Verification items for the finished model (mm, model axes). Face numbers are marked on the shaded views. A direction names the side the tool comes from. Round coordinates to 2 decimals unless told otherwise and drop trailing zeros. Order: outer loops, then holes, each group sorted by start corner. A loop starts at its lowest first (then second) coordinate and runs counter-clockwise, first axis right, second up. Notation, with made-up numbers: (74, 34) -> (132, 34) arc R31 cw to (132, 65) -> close; hole circle Ø6 at (26, -33). An arc over 180 degrees is marked (long way). Write item = value, one per line. Start each with the question number.
from build123d import *

# Parameters (mm, degrees)
SKETCH1_W                  = 68.6
SKETCH1_H                  = 20.38979341
BRACKETBASE_DEPTH          = 5
SKETCH2_W                  = 20.38979341
SKETCH2_H                  = 12
LEGMOUNTINGTAB_DEPTH       = 5
SKETCH3_R                  = 2
LEGMOUNTINGHOLES_DEPTH     = 5
SKETCH4_W                  = 20.38979341
SKETCH4_H                  = 7
ARDUINOMOUNTINGTAB_DEPTH   = 4.38979341
SKETCH5_R                  = 2
ARDUINOMOUNTINGHOLES_DEPTH = 5
FILLET1_R                  = 2


with BuildPart() as part:
    # Sketch1 → bracketBase (new body)
    with BuildSketch(Plane(origin=(0, 0, 0), x_dir=(1, 0, 0), z_dir=(0, 1, 0))):
        with Locations((34.3, 10.194896705)):
            Rectangle(SKETCH1_W, SKETCH1_H)
    extrude(amount=BRACKETBASE_DEPTH)

    # Sketch2 → legMountingTab (add)
    with BuildSketch(Plane.ZY):
        with Locations((-10.194896705, 6)):
            Rectangle(SKETCH2_W, SKETCH2_H)
    legmountingtab = extrude(amount=-LEGMOUNTINGTAB_DEPTH)

    # Sketch3 → legMountingHoles (cut)
    with BuildSketch(Plane(origin=(5, 0, 0), x_dir=(0, 0, -1), z_dir=(1, 0, 0))):
        with Locations((15.13979341, 8.75)):
            Circle(SKETCH3_R)
        with Locations((5.13979341, 8.75)):
            Circle(SKETCH3_R)
    legmountingholes = extrude(amount=-LEGMOUNTINGHOLES_DEPTH, mode=Mode.SUBTRACT)

    # legMountingHoles2: legMountingTab, legMountingHoles across plane
    add(legmountingtab.mirror(Plane.ZY.offset(-34.3)))
    add(legmountingholes.mirror(Plane.ZY.offset(-34.3)), mode=Mode.SUBTRACT)

    # Sketch4 → arduinoMountingTab (add)
    with BuildSketch(Plane.XY):
        with Locations((34.3, -3.5)):
            Rectangle(SKETCH4_W, SKETCH4_H)
    extrude(amount=-ARDUINOMOUNTINGTAB_DEPTH)

    # Sketch5 → arduinoMountingHoles (cut)
    with BuildSketch(Plane.XY):
        with Locations((39.397448352, -3.5)):
            Circle(SKETCH5_R)
        with Locations(Location((29.202551647, -3.5, 0), (0, 0, 180))):
            Circle(SKETCH5_R)
    extrude(amount=-ARDUINOMOUNTINGHOLES_DEPTH, mode=Mode.SUBTRACT)

    # Fillet1
    fillet1_edges = [part.edges().sort_by_distance(p)[0] for p in [
        (44.494896705, 0, -2.194896705),
        (44.494896705, -7, -2.194896705),
        (24.105103295, -7, -2.194896705),
        (24.105103295, 0, -2.194896705),
    ]]
    fillet(fillet1_edges, radius=FILLET1_R)


solid = part.part
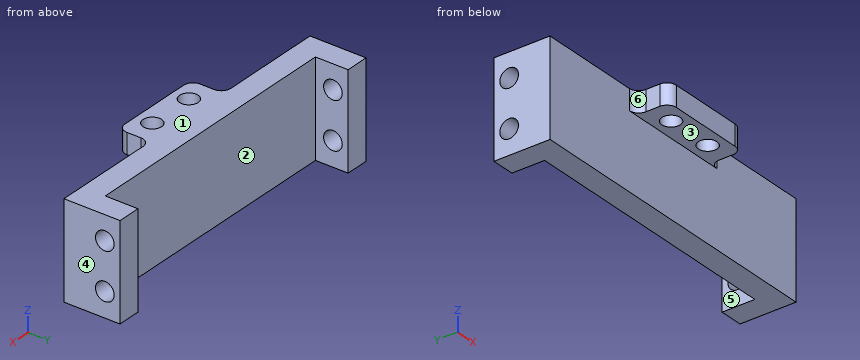
(1) Cross-section at A-A (y = 5.75). Enter the section's corners in (x, z).
(2) Cross-section at D-D (x = 29.5). Enter the section's corners in (y, z), and give its area (3 significant figures).
(3) Cross-section at C-C (z = -11.25). Enter the section's corners in (x, y).
(4) Cross-section at B-B (y = -3.5). Enter the section's corners in (x, z), and give its area (3 significant figures).
(5) Set-up check for the marked faces 1, 2 and 3: record each of +Z, -Z, +X, -X, +Y, -Y from which the full face is reachable in a straight line by a thin tool's end or side.
(6) Scan lines: line 1 along X through (y, z) = (11, -4.5); line 2 along Y through (x, z) = (35, -6.75); line 3 along Z through (x, y) = (32.5, -4). Record each from-to range of solid material in increasing order. Write a range as from..to.
(7) Depth check by flat-ended pin: pin 1 (2.5 mm diameter, centred on y = 8.75, z = -5.14, fed in from +X); pin 2 (4.5 mm diameter, centred on x = 39.4, y = -3.5, fed in from -Z); pin 3 (2.5 mm diameter, centred on y = -3, z = -2.5, fed in from +X); pin 4 (2 mm diameter, centred on x = 26, z = -8, fed in from -Y). Enter the tip coordinate at first touch or a pass-through.
(8) Draft check along X on the marked faces 4, 5 and 6. Enter one of: +X half, -X half, draft (parallel to the pull), parting line (faces both ways), or undercut.
Outcome:
q1.outline = (0, -20.39) -> (5, -20.39) -> (5, 0) -> (0, 0) -> close; (63.6, -20.39) -> (68.6, -20.39) -> (68.6, 0) -> (63.6, 0) -> close
q2.outline = (-7, -4.39) -> (-5.48, -4.39) -> (-5.48, 0) -> (-7, 0) -> close; (-1.52, -4.39) -> (0, -4.39) -> (0, -20.39) -> (5, -20.39) -> (5, 0) -> (-1.52, 0) -> close
q2.area = 115 mm^2
q3.outline = (0, 0) -> (68.6, 0) -> (68.6, 12) -> (63.6, 12) -> (63.6, 5) -> (5, 5) -> (5, 12) -> (0, 12) -> close
q4.outline = (24.11, -4.39) -> (27.2, -4.39) -> (27.2, 0) -> (24.11, 0) -> close; (31.2, -4.39) -> (37.4, -4.39) -> (37.4, 0) -> (31.2, 0) -> close; (41.4, -4.39) -> (44.49, -4.39) -> (44.49, 0) -> (41.4, 0) -> close
q4.area = 54.4 mm^2
q5.face_1 = +Z, +X, -X, +Y, -Y
q5.face_2 = +Z, -Z, +Y
q5.face_3 = -Z, +X, -X, -Y
q6.line_1 = 0..5, 63.6..68.6
q6.line_2 = 0..5
q6.line_3 = -4.39..0
q7.pin_1 = through
q7.pin_2 = -4.39
q7.pin_3 = 44.51
q7.pin_4 = 0
q8.face_4 = +X half
q8.face_5 = undercut
q8.face_6 = -X half
